```python
from build123d import *

# Parameters (mm, degrees)
SKETCH_1_W          = 135
SKETCH_1_H          = 40
EXTRUDE_1_DEPTH     = 4
SKETCH_2_W          = 20
SKETCH_2_H          = 20
CUT_EXTRUDE_1_DEPTH = 71.514182971
FILLET_1_R          = 4
SKETCH_3_R          = 1.5
CUT_EXTRUDE_2_DEPTH = 71.514182971
SKETCH_4_R          = 1.5
CUT_EXTRUDE_3_DEPTH = 71.514182971


with BuildPart() as part:
    # 草图1 → 凸台-拉伸1 (new body)
    with BuildSketch(Plane.XY):
        Rectangle(SKETCH_1_W, SKETCH_1_H)
    extrude(amount=EXTRUDE_1_DEPTH)

    # 草图2 → 切除-拉伸1 (cut, through all)
    with BuildSketch(Plane.XY.offset(4)):
        with Locations((-57.5, 10)):
            Rectangle(SKETCH_2_W, SKETCH_2_H)
        with Locations((57.5, 10)):
            Rectangle(SKETCH_2_W, SKETCH_2_H)
    extrude(amount=-CUT_EXTRUDE_1_DEPTH, mode=Mode.SUBTRACT)

    # 圆角1
    fillet_1_edges = [part.edges().sort_by_distance(p)[0] for p in [
        (-47.5, 0, 2),
        (47.5, 0, 2),
    ]]
    fillet(fillet_1_edges, radius=FILLET_1_R)

    # 草图3 → 切除-拉伸2 (cut, through all)
    with BuildSketch(Plane.XY.offset(4)):
        with Locations((0, 12.5)):
            Circle(SKETCH_3_R)
        with Locations((-30, 12.5)):
            Circle(SKETCH_3_R)
        with Locations(Location((30, 12.5, 0), (0, 0, 180))):
            Circle(SKETCH_3_R)
    extrude(amount=-CUT_EXTRUDE_2_DEPTH, mode=Mode.SUBTRACT)

    # 草图4 → 切除-拉伸3 (cut, through all)
    with BuildSketch(Plane.XY.offset(4)):
        with Locations((-41.75, -13.5)):
            Circle(SKETCH_4_R)
        with Locations((-33.75, -13.5)):
            Circle(SKETCH_4_R)
        with Locations(Location((33.75, -13.5, 0), (0, 0, 180))):
            Circle(SKETCH_4_R)
        with Locations(Location((41.75, -13.5, 0), (0, 0, 180))):
            Circle(SKETCH_4_R)
    extrude(amount=-CUT_EXTRUDE_3_DEPTH, mode=Mode.SUBTRACT)


solid = part.part
```
Source: CAD feature listing. Evaluate the final solid. Frame: model axes, mm. A direction names the side the tool comes from. Round coordinates to 2 decimals unless told otherwise and drop trailing zeros. Loops run counter-clockwise (first coordinate to the right, second up) from the corner with the lowest first, then second, coordinate; pieces in that order, holes last. Notation, with made-up numbers: M -36,-30 L 4,-30 A28 ccw 4,-10 Z; hole C 53.5,2 d5. An arc over 180 degrees is marked long. Use a Markdown table: item, result. Add a question column.
1. Section query D-D on x = 59.5. Return the cut outline in (y, z).
2. Section query B-B on x = 41.75. Return the cut outline in (y, z).
3. Mould query, pull axis X, two halves, no side actions, for faces 1 (the cylindrical face through (31.5, 12.43, 2.03)), 2 (the cylindrical face through (48.641, 1.203, 1.972)), 3 (the cylindrical face through (-34.94, -14.41, 2.03)), 4 (the flat face through (-1, 0, 4)). Classes: pulls with the +X half, pulls with the -X half, needs draft (parallel to the pull), parting line crosses it, or undercut.
4. Section query C-C on z = 2.95. Return the cut outline in (x, y), then the cut area to 3 significant figures.
5. Reachability of faces 5 (the flat face through (-60, 0, 2)), 6 (the flat face through (47.5, 12, 2)), 7 (the flat face through (-1, 0, 0)) from +Z, -Z, +X, -X, +Y, -Y: full face, straight path, thin tool, end or side. Return the list, or none.
6. Section query A-A on y = 12.5. Return the cut outline in (x, z), then the cut area to 3 significant figures.
7. Line query: line 1 (Y direction, x = 0, z = 2.5); line 2 (Y direction, x = -41.75, z = 0.95); line 3 (X direction, y = 13.5, z = 2.7). Output: solid intervals per line, ascending.
8. Contact query for flat-ended pins moving along their axis: P1, Ø2, axis at x = -57, z = 2.5, coming from the +Y side; P2, Ø2, axis at y = 6.5, z = 1, coming from the -X side; P3, Ø3, axis at x = -30, y = 3, coming from the -Z side. Output: stop coordinate, or through.
Reported:
| question | item | result |
|---|---|---|
| 1 | outline | M -20,0 L 0,0 L 0,4 L -20,4 Z |
| 2 | outline | M -20,0 L -15,0 L -15,4 L -20,4 Z; M -12,0 L 20,0 L 20,4 L -12,4 Z |
| 3 | face 1 | undercut |
| 3 | face 2 | pulls with the +X half |
| 3 | face 3 | undercut |
| 3 | face 4 | needs draft |
| 4 | outline | M -67.5,-20 L 67.5,-20 L 67.5,0 L 51.5,0 A4 cw 47.5,4 L 47.5,20 L -47.5,20 L -47.5,4 A4 cw -51.5,0 L -67.5,0 Z; hole C -41.75,-13.5 d3; hole C -33.75,-13.5 d3; hole C -30,12.5 d3; hole C 0,12.5 d3; hole C 30,12.5 d3; hole C 33.75,-13.5 d3; hole C 41.75,-13.5 d3 |
| 4 | area | 4,560 mm² |
| 5 | face 5 | +Z, -Z, -X, +Y |
| 5 | face 6 | +Z, -Z, +X, +Y |
| 5 | face 7 | -Z, +X, -X, +Y, -Y |
| 6 | outline | M -47.5,0 L -31.5,0 L -31.5,4 L -47.5,4 Z; M -28.5,0 L -1.5,0 L -1.5,4 L -28.5,4 Z; M 1.5,0 L 28.5,0 L 28.5,4 L 1.5,4 Z; M 31.5,0 L 47.5,0 L 47.5,4 L 31.5,4 Z |
| 6 | area | 344 mm² |
| 7 | line 1 | y = -20 to 11, 14 to 20 |
| 7 | line 2 | y = -20 to -15, -12 to 20 |
| 7 | line 3 | x = -47.5 to -31.12, -28.88 to -1.12, 1.12 to 28.88, 31.12 to 47.5 |
| 8 | P1 | stops at y = 0 |
| 8 | P2 | stops at x = -47.5 |
| 8 | P3 | stops at z = 0 |
